For this review, take the finished solid that the model builds, in its own axes (mm). A direction names the side the tool comes from. Round coordinates to 2 decimals unless told otherwise and drop trailing zeros. Write each loop counter-clockwise with the first axis right and the second up, starting at its lowest first coordinate (ties: lowest second). Pieces come first, ordered by that corner, then holes.
from build123d import *

# Parameters (mm, degrees)
SKETCH1_W           = 70
SKETCH1_H           = 70
BOSS_EXTRUDE1_DEPTH = 2
SKETCH2_W           = 2
SKETCH2_H           = 20
BOSS_EXTRUDE2_DEPTH = 2
SKETCH3_W           = 20
SKETCH3_H           = 2
CUT_EXTRUDE1_DEPTH  = 2
SKETCH4_W           = 12.53
SKETCH4_H           = 7.1
CUT_EXTRUDE2_DEPTH  = 10


with BuildPart() as part:
    # Sketch1 → Boss-Extrude1 (new body)
    with BuildSketch(Plane.XY):
        Rectangle(SKETCH1_W, SKETCH1_H)
    extrude(amount=-BOSS_EXTRUDE1_DEPTH)

    # Sketch2 → Boss-Extrude2 (add)
    with BuildSketch(Plane.XY):
        with Locations((-36, 15)):
            Rectangle(SKETCH2_W, SKETCH2_H)
        with Locations((-36, -15)):
            Rectangle(SKETCH2_W, SKETCH2_H)
        with Locations((36, -15)):
            Rectangle(SKETCH2_W, SKETCH2_H)
        with Locations((36, 15)):
            Rectangle(SKETCH2_W, SKETCH2_H)
    extrude(amount=-BOSS_EXTRUDE2_DEPTH)

    # Sketch3 → Cut-Extrude1 (cut)
    with BuildSketch(Plane.XY):
        with Locations((-15, 34)):
            Rectangle(SKETCH3_W, SKETCH3_H)
        with Locations((15, 34)):
            Rectangle(SKETCH3_W, SKETCH3_H)
        with Locations((-15, -34)):
            Rectangle(SKETCH3_W, SKETCH3_H)
        with Locations((15, -34)):
            Rectangle(SKETCH3_W, SKETCH3_H)
    extrude(amount=-CUT_EXTRUDE1_DEPTH, mode=Mode.SUBTRACT)

    # Sketch4 → Cut-Extrude2 (cut)
    with BuildSketch(Plane.XY):
        Rectangle(SKETCH4_W, SKETCH4_H)
    extrude(amount=-CUT_EXTRUDE2_DEPTH, mode=Mode.SUBTRACT)


solid = part.part
(1) For faces 1 (the face through (5, -34, -1)), 2 (the face through (36, 25, -1)), 3 (the face through (36, 5, -1)), list the 3-axis set-ups (+Z, -Z, +X, -X, +Y, -Y) from which the entire face can be reached by the end or side of a thin tool; tool diameter is ignored.
Geometry check:
face 1: +Z, -Z, -Y
face 2: +Z, -Z, +X, +Y
face 3: +Z, -Z, +X
(2) Mouldability with a two-part tool opening along Y and no side actions: class faces 4 (the face through (37, -15, -1)), 5 (the face through (-36, 5, -1)), 6 (the face through (36, -25, -1)) as pulls with the +Y half, pulls with the -Y half, needs draft (parallel to the pull), parting line crosses it, or undercut.
Geometry check:
face 4: needs draft
face 5: undercut
face 6: pulls with the -Y half
(3) We need section A-A, the plane x = 3. Give the boundary of the cut face in (y, z).
Geometry check:
outline: (-35, -2) - (-3.55, -2) - (-3.55, 0) - (-35, 0) - close; (3.55, -2) - (35, -2) - (35, 0) - (3.55, 0) - close
(4) For line 1 along X through (y, z) = (-1.5, -1.9) (3 decimals); line 2 along Y through (x, z) = (3, -0.1); line 3 along X through (y, z) = (26, -0.05), list the stretches that pass through material, from the lowest coordinate up.
Geometry check:
line 1: x = -35 to -6.265, 6.265 to 35
line 2: y = -35 to -3.55, 3.55 to 35
line 3: x = -35 to 35
(5) For pin 1 Ø1 at (y, z) = (-34, -1) entering from -X; pin 2 Ø0.6 at (x, z) = (36.5, -1) entering from -Y; pin 3 Ø1 at (y, z) = (-34, -1) entering from +X, all flat-tipped, find the tip position at first contact; note any pin that passes through.
Geometry check:
pin 1: stops at x = -35
pin 2: stops at y = -25
pin 3: stops at x = 35
(6) We need section C-C, the plane y = -27.5. Give the boundary of the cut face in (x, z), and give its area (3 significant figures).
Geometry check:
outline: (-35, -2) - (35, -2) - (35, 0) - (-35, 0) - close
area: 140 mm2
(7) We need section B-B, the plane x = 13. Give the boundary of the cut face in (y, z).
Geometry check:
outline: (-33, -2) - (33, -2) - (33, 0) - (-33, 0) - close
